from build123d import *

# Parameters (mm, degrees)
F0_W           = 40
F0_H           = 8
F2_DEPTH       = 1
F1_R           = 3.5
F3_DEPTH       = 3
F4_R           = 7.5
F5_DEPTH       = 4
F6_R           = 4
F7_R           = 5
F9_D           = 11
F9_CBORE_D     = 13.25
F9_CBORE_DEPTH = 7
F12_D          = 6
F13_R          = 2


with BuildPart() as f2:
    # F0 (on Top) → F2 (new body, symmetric)
    with BuildSketch(Plane.XY):
        Rectangle(F0_W, F0_H)
    extrude(amount=F2_DEPTH, both=True)

    # F1 (on face) → F3 (join)
    with BuildSketch(Plane.XY):
        with Locations((-15.75, 0)):
            Circle(F1_R)
        with Locations((15.75, 0)):
            Circle(F1_R)
    extrude(amount=F3_DEPTH)

    # F4 (on Front) → F5 (join, symmetric)
    with BuildSketch(Plane.XZ):
        with Locations((0, 8)):
            Circle(F4_R)
    extrude(amount=F5_DEPTH, both=True)

    # F6
    f6_edges = [f2.edges().sort_by_distance(p)[0] for p in [
        (2.692582, 0, 1),
    ]]
    fillet(f6_edges, radius=F6_R)

    # F7
    f7_edges = [f2.edges().sort_by_distance(p)[0] for p in [
        (-2.692582, 0, 1),
    ]]
    fillet(f7_edges, radius=F7_R)

    # F9 (through all)
    with Locations(Plane.XZ.offset(4)):
        with Locations((0, 8)):
            CounterBoreHole(F9_D / 2, F9_CBORE_D / 2, F9_CBORE_DEPTH)

    # F12 (through all)
    with Locations(Plane.XY.offset(3)):
        with Locations((15.75, 0), (-15.75, 0)):
            Hole(F12_D / 2)

    # F13
    f13_edges = [f2.edges().sort_by_distance(p)[0] for p in [
        (-20, -4, 0),
        (-20, 4, 0),
        (20, 4, 0),
        (20, -4, 0),
    ]]
    fillet(f13_edges, radius=F13_R)


solid = f2.part
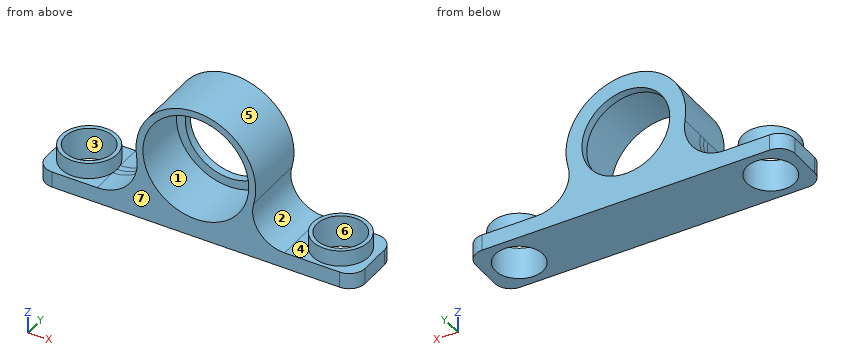
Could you check a few things on this model? Use its own coordinates, in mm. Face numbers are marked on the shaded views. A direction names the side the tool comes from. Coordinates: 2 decimals unless noted, no trailing zeros. Loops run counter-clockwise (first coordinate to the right, second up) from the corner with the lowest first, then second, coordinate; pieces in that order, holes last. Notation, with made-up numbers: (-29, 14.5) -> (9, 14.5) arc R11 cw to (9, 34.5) -> close; hole circle Ø5 at (65.25, 75.5). An arc over 180 degrees is marked (long way). Answer in a Markdown table with one row per item.
(1) For the marked faces 1, 2, 3 and 4, which set-ups out of +Z, -Z, +X, -X, +Y, -Y let a thin tool reach every point of the face, with its end or its side?
Results found:
| item | result |
|---|---|
| face 1 | -Y |
| face 2 | +Y, -Y |
| face 3 | +Z, -Z |
| face 4 | +Z |
(2) If I drill on probe 1 along Y at (x, z) = (15.75, 1.8); probe 2 along X at (y, z) = (-3, 10); probe 3 along Z at (x, y) = (5, -1.5), over which ranges is the centre line in solid material (lowest first)?
Results found:
| item | result |
|---|---|
| probe 1 | y = -3.5 to -3, 3 to 3.5 |
| probe 2 | x = -7.23 to -6.32, 6.32 to 7.23 |
| probe 3 | z = -1 to 3.65, 12.35 to 13.59 |
(3) Thinking about a two-plate mould opening in X: for the marked faces 5, 6 and 7, which applies, released by +X, released by -X, zero draft, split by the parting line, or undercut?
Results found:
| item | result |
|---|---|
| face 5 | split by the parting line |
| face 6 | undercut |
| face 7 | zero draft |
(4) Will these pins go through, and if not, where does the flat tip stop? pin 1 Ø2.5 at (x, y) = (-17.5, 1) entering from +Z; pin 2 Ø2 at (x, y) = (3.5, 2) entering from +Z; pin 3 Ø1.5 at (x, y) = (7, 0.5) entering from +Z.
Results found:
| item | result |
|---|---|
| pin 1 | stops at z = 3 |
| pin 2 | stops at z = 15.07 |
| pin 3 | stops at z = 12.15 |
(5) Imagine slicing it at B-B (z = 11.25). List the corners of the cut face in (x, y) for me.
Results found:
| item | result |
|---|---|
| outline | (-6.76, -4) -> (-5.77, -4) -> (-5.77, 3) -> (-4.44, 3) -> (-4.44, 4) -> (-6.76, 4) -> close; (4.44, 3) -> (5.77, 3) -> (5.77, -4) -> (6.76, -4) -> (6.76, 4) -> (4.44, 4) -> close |
(6) Imagine slicing it at A-A (x = -15.75). List the corners of the cut face in (y, z) for me, plus the area to 3 significant figures.
Results found:
| item | result |
|---|---|
| outline | (-4, -1) -> (-3, -1) -> (-3, 3) -> (-3.5, 3) -> (-3.5, 1) -> (-4, 1) -> close; (3, -1) -> (4, -1) -> (4, 1) -> (3.5, 1) -> (3.5, 3) -> (3, 3) -> close |
| area | 6.00 mm^2 |
(7) Imagine slicing it at C-C (x = 6). List the corners of the cut face in (y, z) for me, plus the area to 3 significant figures.
Results found:
| item | result |
|---|---|
| outline | (-4, -1) -> (4, -1) -> (4, 12.5) -> (-4, 12.5) -> (-4, 10.81) -> (3, 10.81) -> (3, 5.19) -> (-4, 5.19) -> close |
| area | 68.7 mm^2 |
